Here's how the part is built. I have some questions about the finished solid (model axes, mm). Face numbers are marked on the shaded views. A direction names the side the tool comes from. Round coordinates to 2 decimals unless told otherwise and drop trailing zeros. Loops run counter-clockwise (first coordinate to the right, second up) from the corner with the lowest first, then second, coordinate; pieces in that order, holes last. Notation, with made-up numbers: M 13.25,-3 L 72.25,-3 A17 cw 72.25,23 Z; hole C 88.25,-8.75 d6. An arc over 180 degrees is marked long. One line per question, with ' | ' between items. Start each with the question number.
```python
from build123d import *

# Parameters (mm, degrees)
SKETCH_1_R                  = 20.4
SKETCH_1_R_2                = 11
EXTRUDE_1_DEPTH             = 5
M3X0_51_D                   = 2.5
HOLE_WIZARD_M31_D           = 3.4
HOLE_WIZARD_M31_CBORE_D     = 6.5
HOLE_WIZARD_M31_CBORE_DEPTH = 3


with BuildPart() as part:
    # Эскиз1 → Бобышка-Вытянуть1 (new body)
    with BuildSketch(Plane(origin=(0, 0, 0), x_dir=(1, 0, 0), z_dir=(0, 1, 0))):
        Circle(SKETCH_1_R)
        Circle(SKETCH_1_R_2, mode=Mode.SUBTRACT)
    extrude(amount=EXTRUDE_1_DEPTH)

    # Отверстие обработанное метчиком M3x0.51 (through all)
    with Locations(Plane(origin=(0, 5, 0), x_dir=(1, 0, 0), z_dir=(0, 1, 0))):
        with Locations((-18.25, 0), (0, 18.25), (18.25, 0), (0, -18.25)):
            Hole(M3X0_51_D / 2)

    # Цековка для винта с внутренним шестигранником M31 (through all)
    with Locations(Plane(origin=(0, 0, 0), x_dir=(-1, 0, 0), z_dir=(0, -1, 0))):
        with Locations((10.606601718, -10.606601718), (-10.606601718, -10.606601718), (-10.606601718, 10.606601718), (10.606601718, 10.606601718)):
            CounterBoreHole(HOLE_WIZARD_M31_D / 2, HOLE_WIZARD_M31_CBORE_D / 2, HOLE_WIZARD_M31_CBORE_DEPTH)


solid = part.part
```
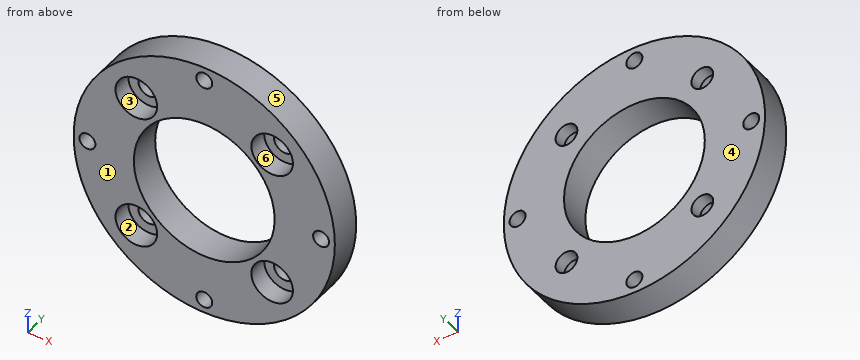
1) We'd pull the mould along Z, two halves only. Please class the marked faces 3, 4, 5 and 6: pulls with the +Z half, pulls with the -Z half, needs draft (parallel to the pull), parting line crosses it, or undercut.
2) I'm going to push flat-ended pins straight in: pin 1 Ø1 at (x, y) = (-11, 0.5) entering from +Z; pin 2 Ø3 at (x, z) = (-10.5, 9.5) entering from -Y; pin 3 Ø2 at (y, z) = (4, -6) entering from -X. Where does each tip first touch, or does it pass through?
3) Please list where these lines run through material, in increasing order: L1, parallel to Z at x = 0, y = 1.35; L2, parallel to Z at x = 12.5, y = 1.9; L3, parallel to Z at x = 17.5, y = 4.2. Write a range as from..to.
4) For the marked faces 1 and 2, which set-ups out of +Z, -Z, +X, -X, +Y, -Y let a thin tool reach every point of the face, with its end or its side?
5) Imagine slicing it at C-C (y = 3.6). State how many separate pieces and enclosed holes the cut face has, then the cut area to 3 significant figures.
6) Imagine slicing it at D-D (x = 18.25). Write out the boundary of the cut face in (y, z), then the cut area to 3 significant figures.
7) Imagine slicing it at B-B (x = 0). Write out the boundary of the cut face in (y, z).
8) Imagine slicing it at A-A (z = 0). Write out the boundary of the cut face in (x, y), then the cut area to 3 significant figures.
Results are:
1) face 3: undercut | face 4: needs draft | face 5: parting line crosses it | face 6: undercut
2) pin 1: z = 17.49 | pin 2: y = 3 | pin 3: x = -19.78
3) L1: -20.4..-19.5, -17..-11, 11..17, 19.5..20.4 | L2: -16.12..-13.25, -7.97..7.97, 13.25..16.12 | L3: -10.48..-1, 1..10.48
4) face 1: +Z, -Z, +X, -X, -Y | face 2: -Y
5) separate pieces: 1 | enclosed holes: 9 | area: 871 mm²
6) outline: M 0,-9.12 L 5,-9.12 L 5,-1.25 L 0,-1.25 Z; M 0,1.25 L 5,1.25 L 5,9.12 L 0,9.12 Z | area: 78.7 mm²
7) outline: M 0,-20.4 L 5,-20.4 L 5,-19.5 L 0,-19.5 Z; M 0,-17 L 5,-17 L 5,-11 L 0,-11 Z; M 0,11 L 5,11 L 5,17 L 0,17 Z; M 0,19.5 L 5,19.5 L 5,20.4 L 0,20.4 Z
8) outline: M -20.4,0 L -19.5,0 L -19.5,5 L -20.4,5 Z; M -17,0 L -11,0 L -11,5 L -17,5 Z; M 11,0 L 17,0 L 17,5 L 11,5 Z; M 19.5,0 L 20.4,0 L 20.4,5 L 19.5,5 Z | area: 69.0 mm²
